Geometry check sheet. Reference: the model listing, model coordinates, mm. Face numbers are marked on the shaded views. A direction names the side the tool comes from. Give positions to 0.01 mm unless a question says otherwise; leave off trailing zeros. Loops run counter-clockwise (first coordinate to the right, second up) from the corner with the lowest first, then second, coordinate; pieces in that order, holes last. Notation, with made-up numbers: (-26, 6.25) - (31, 6.25) arc R33 ccw to (31, 34.25) - close; hole circle Ø2 at (-23, 53). An arc over 180 degrees is marked (long way). One line per question, with ' | ' between items. Start each with the question number.
from build123d import *

# Parameters (mm, degrees)
EXTRU_MINCE1_DEPTH      = 60
BOSS_EXTRU_1_START      = 1
BOSS_EXTRU_1_DEPTH      = 1
BOSS_EXTRU_2_DEPTH      = 1
ESQUISSE4_W             = 166
ESQUISSE4_H             = 210
ESQUISSE4_W_2           = 106
ESQUISSE4_H_2           = 93
ESQUISSE4_H_3           = 38
BOSS_EXTRU_3_DEPTH      = 5
ESQUISSE5_R             = 2.5
ENL_V_MAT_EXTRU_1_DEPTH = 166.924681708


with BuildPart() as part:
    # Esquisse1 → Extru.-Mince1 (new, symmetric)
    with BuildSketch(Plane(origin=(0, 0, 0), x_dir=(0, 0, -1), z_dir=(1, 0, 0))):
        with BuildLine():
            ThreePointArc((0, -54), (46.554240379, -27.362432324), (47.179157474, 26.27027027))
            Line((47.179157474, 26.27027027), (0, 111))
            Line((0, 111), (-0.873688101, 110.513513514))
            Line((-0.873688101, 110.513513514), (46.305469372, 25.783783784))
            ThreePointArc((46.305469372, 25.783783784), (45.692124817, -26.855720615), (0, -53))
            Line((0, -53), (0, -54))
        make_face()
    extrude(amount=EXTRU_MINCE1_DEPTH, both=True)

    # Esquisse2 → Boss.-Extru.1 (add)
    with BuildSketch(Plane(origin=(60, 0, 0), x_dir=(0, 0, -1), z_dir=(1, 0, 0)).offset(BOSS_EXTRU_1_START)):
        with BuildLine():
            Line((0, 111), (0, -54))
            ThreePointArc((0, -54), (46.554240379, -27.362432324), (47.179157474, 26.27027027))
            Line((47.179157474, 26.27027027), (0, 111))
        make_face()
    extrude(amount=-BOSS_EXTRU_1_DEPTH)

    # Esquisse3 → Boss.-Extru.2 (add)
    with BuildSketch(Plane.ZY.offset(60)):
        with BuildLine():
            Line((0, 111), (0, -54))
            ThreePointArc((0, -54), (-46.554240379, -27.362432324), (-47.179157474, 26.27027027))
            Line((-47.179157474, 26.27027027), (0, 111))
        make_face()
    extrude(amount=BOSS_EXTRU_2_DEPTH)

    # Esquisse4 → Boss.-Extru.3 (add)
    with BuildSketch(Plane.XY):
        with Locations((0, 26)):
            Rectangle(ESQUISSE4_W, ESQUISSE4_H)
        with Locations((0, 58.5)):
            Rectangle(ESQUISSE4_W_2, ESQUISSE4_H_2, mode=Mode.SUBTRACT)
        with Locations((0, -34)):
            Rectangle(ESQUISSE4_W_2, ESQUISSE4_H_3, mode=Mode.SUBTRACT)
    extrude(amount=BOSS_EXTRU_3_DEPTH)

    # Esquisse5 → Enlèv. mat.-Extru.1 (cut, through all)
    with BuildSketch(Plane.XY.offset(5)):
        with Locations((-70, 115)):
            Circle(ESQUISSE5_R)
        with Locations((-70, 26)):
            Circle(ESQUISSE5_R)
        with Locations((-70, -63)):
            Circle(ESQUISSE5_R)
        with Locations((70, -63)):
            Circle(ESQUISSE5_R)
        with Locations((70, 26)):
            Circle(ESQUISSE5_R)
        with Locations((70, 115)):
            Circle(ESQUISSE5_R)
    extrude(amount=-ENL_V_MAT_EXTRU_1_DEPTH, mode=Mode.SUBTRACT)


solid = part.part
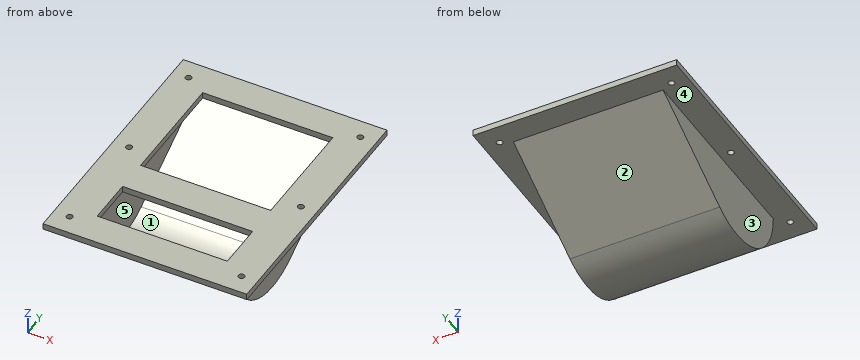
(1) Depth check by flat-ended pin: pin 1 Ø2 at (x, y) = (17, -36.5) entering from +Z; pin 2 Ø5 at (x, z) = (36, -33) entering from +Y; pin 3 Ø10 at (y, z) = (-57.5, -24) entering from -X; pin 4 Ø10 at (x, z) = (-51.5, -32.5) entering from +Y. Enter the tip coordinate at first touch or a pass-through.
(2) Mould release check, pull along X, two halves, no side actions. Record for the marked faces 3, 4 and 5: pulls with the +X half, pulls with the -X half, needs draft (parallel to the pull), parting line crosses it, or undercut.
(3) Section check C-C, the plane x = 21. Record the boundary of the cut face in (y, z), and give its area (3 significant figures).
(4) Section check B-B, the plane y = 115. Record the boundary of the cut face in (x, z), and give its area (3 significant figures).
(5) Tool access check on the marked faces 1 and 2. Record the directions out of +Z, -Z, +X, -X, +Y, -Y that give a thin tool (end or side, any length) a straight path to the whole face; none if there is none.
(6) Section check D-D, the plane z = -17. Record the boundary of the cut face in (x, y).
(7) Material ranges on line 1 (Y direction, x = 70, z = 2); line 2 (X direction, y = 40, z = -31.5); line 3 (Z direction, x = 63.5, y = 22), recorded low to high.
(8) Section check A-A, the plane x = 70. Record the boundary of the cut face in (y, z), and give its area (3 significant figures).
Numbers:
1) pin 1: z = -37.45 | pin 2: y = 56.22 | pin 3: through | pin 4: y = 61.61
2) face 3: pulls with the -X half | face 4: needs draft | face 5: undercut
3) outline: (-79, 0) - (-54, 0) arc R54 ccw to (26.27, -47.18) - (111, 0) - (131, 0) - (131, 5) - (105, 5) - (105, 0) - (108.94, 0) - (25.78, -46.31) arc R53 cw to (-53, 0) - (-53, 5) - (-79, 5) - close; (-15, 0) - (12, 0) - (12, 5) - (-15, 5) - close | area: 602 mm^2
4) outline: (-83, 0) - (-72.5, 0) - (-72.5, 5) - (-83, 5) - close; (-67.5, 0) - (67.5, 0) - (67.5, 5) - (-67.5, 5) - close; (72.5, 0) - (83, 0) - (83, 5) - (72.5, 5) - close | area: 780 mm^2
5) face 1: none | face 2: -Z, +X, -X, +Y
6) outline: (-61, -51.25) - (61, -51.25) - (61, 80.47) - (-61, 80.47) - close; hole (-60, -50.2) - (60, -50.2) - (60, 78.41) - (-60, 78.41) - close
7) line 1: -79 to -65.5, -60.5 to 23.5, 28.5 to 112.5, 117.5 to 131 | line 2: -61 to -60, 60 to 61 | line 3: 0 to 5
8) outline: (-79, 0) - (-65.5, 0) - (-65.5, 5) - (-79, 5) - close; (-60.5, 0) - (23.5, 0) - (23.5, 5) - (-60.5, 5) - close; (28.5, 0) - (112.5, 0) - (112.5, 5) - (28.5, 5) - close; (117.5, 0) - (131, 0) - (131, 5) - (117.5, 5) - close | area: 975 mm^2
